Here's how the part is built. I have some questions about the finished solid (model axes, mm). A direction names the side the tool comes from. Give positions to 0.01 mm unless a question says otherwise; leave off trailing zeros. Order: outer loops, then holes, each group sorted by start corner. A loop starts at its lowest first (then second) coordinate and runs counter-clockwise, first axis right, second up. Notation, with made-up numbers: (-13.75, -12.75) - (36.25, -12.75) arc R30 ccw to (36.25, 11.25) - close; hole circle Ø4 at (40.25, 58.5). An arc over 180 degrees is marked (long way). One line per question, with ' | ' between items.
from build123d import *

# Parameters (mm, degrees)
BOSS_EXTRUDE1_DEPTH  = 3.175
M5_CLEARANCE_HOLE1_D = 5.3
BOSS_EXTRUDE2_DEPTH  = 3.175
M5_CLEARANCE_HOLE2_D = 5.3
M4_CLEARANCE_HOLE1_D = 4.3
M2_CLEARANCE_HOLE1_D = 2.2


with BuildPart() as part:
    # Sketch1 → Boss-Extrude1 (new body)
    with BuildSketch(Plane.XY):
        with BuildLine():
            Line((-79, 10), (79, 10))
            ThreePointArc((79, 10), (89, 0), (79, -10))
            Line((79, -10), (-79, -10))
            ThreePointArc((-79, -10), (-89, 0), (-79, 10))
        make_face()
    extrude(amount=BOSS_EXTRUDE1_DEPTH)

    # M5 Clearance Hole1 (through all)
    with Locations(Plane(origin=(0, 0, 0), x_dir=(-1, 0, 0), z_dir=(0, 0, -1))):
        with Locations((-79, 0), (79, 0)):
            Hole(M5_CLEARANCE_HOLE1_D / 2)

    # Sketch8 → Boss-Extrude2 (add)
    with BuildSketch(Plane(origin=(0, 0, 0), x_dir=(-1, 0, 0), z_dir=(0, 0, -1))):
        Polygon((38, 10), (36.129310345, 17.75), (-17.25, 17.75), (-17.25, 10), align=None)
    extrude(amount=-BOSS_EXTRUDE2_DEPTH)

    # M5 Clearance Hole2 (through all)
    with Locations(Plane(origin=(0, 0, 0), x_dir=(-1, 0, 0), z_dir=(0, 0, -1))):
        with Locations((7, 13), (29, 13)):
            Hole(M5_CLEARANCE_HOLE2_D / 2)

    # M4 Clearance Hole1 (through all)
    with Locations(Plane(origin=(0, 0, 0), x_dir=(-1, 0, 0), z_dir=(0, 0, -1))):
        with Locations((0, 0), (-55, 0), (18, 13), (65, 0)):
            Hole(M4_CLEARANCE_HOLE1_D / 2)

    # M2 Clearance Hole1 (through all)
    with Locations(Plane(origin=(0, 0, 0), x_dir=(-1, 0, 0), z_dir=(0, 0, -1))):
        with Locations((-18.8375, -2.1), (-18.8375, 2.1)):
            Hole(M2_CLEARANCE_HOLE1_D / 2)


solid = part.part
1) I want a section at B-B (z = 1.2). State how many separate pieces and enclosed holes the cut face has, plus the area to 3 significant figures.
Model answer:
separate pieces: 1 | enclosed holes: 10 | area: 3,740 mm2
2) I want a section at A-A (x = -29). List the corners of the cut face in (y, z) for me (3 decimals), plus the area to 3 significant figures.
Model answer:
outline: (-10, 0) - (10.35, 0) - (10.35, 3.175) - (-10, 3.175) - close; (15.65, 0) - (17.75, 0) - (17.75, 3.175) - (15.65, 3.175) - close | area: 71.3 mm2
3) I want a section at C-C (x = 55). List the corners of the cut face in (y, z) for me (3 decimals), plus the area to 3 significant figures.
Model answer:
outline: (-10, 0) - (-2.15, 0) - (-2.15, 3.175) - (-10, 3.175) - close; (2.15, 0) - (10, 0) - (10, 3.175) - (2.15, 3.175) - close | area: 49.8 mm2
4) I'm going to push flat-ended pins straight in: P1, Ø4, axis at x = -65, y = 0, coming from the +Z side; P2, Ø1, axis at x = -25, y = 1, coming from the -Z side; P3, Ø1, axis at x = 36.5, z = 2, coming from the +Y side. Where does each tip first touch, or does it pass through?
Model answer:
P1: passes through | P2: stops at z = 0 | P3: stops at y = 10
5) On a 3-axis mill with a long thin cutter (end or side, diameter ignored), from which of +Z, -Z, +X, -X, +Y, -Y can I reach the whole of each face in a straight line? I mean faces 1 (the face through (-10, 17.75, 2)), 2 (the face through (17.25, 14, 2)). Say none if no direction works.
Model answer:
face 1: +Z, -Z, +X, -X, +Y | face 2: +Z, -Z, +X, +Y
6) I want a section at D-D (y = 8.5). List the corners of the cut face in (x, z) for me (3 decimals), plus the area to 3 significant figures.
Model answer:
outline: (-84.268, 0) - (84.268, 0) - (84.268, 3.175) - (-84.268, 3.175) - close | area: 535 mm2
7) Please list where these lines run through material, in increasing order: L1, parallel to Y at x = 0, z = 1.95; L2, parallel to Y at x = -18, z = 1.35; L3, parallel to X at y = 10.75, z = 2.95.
Model answer:
L1: y = -10 to -2.15, 2.15 to 17.75 | L2: y = -10 to 10.85, 15.15 to 17.75 | L3: x = -37.82 to -30.4, -27.6 to -8.4, -5.6 to 17.25
8) Thinking about a two-plate mould opening in X: for faces 3 (the face through (-37.078, 13.821, 1.565)), 4 (the face through (-9.103, 11.388, 1.61)), 5 (the face through (-59, 10, 2)), which applies, +X half, -X half, draft (parallel to the pull), parting line (faces both ways), or undercut?
Model answer:
face 3: -X half | face 4: undercut | face 5: draft
